Source: CAD feature listing. Evaluate the final solid. Frame: model axes, mm. Face numbers are marked on the shaded views. A direction names the side the tool comes from. Give positions to 0.01 mm unless a question says otherwise; leave off trailing zeros. Order: outer loops, then holes, each group sorted by start corner. A loop starts at its lowest first (then second) coordinate and runs counter-clockwise, first axis right, second up. Notation, with made-up numbers: (20, 88) - (28, 88) arc R14 ccw to (28, 95) - close; hole circle Ø1 at (15.25, 17.25). An arc over 180 degrees is marked (long way). Answer as CSV lines item,"result".
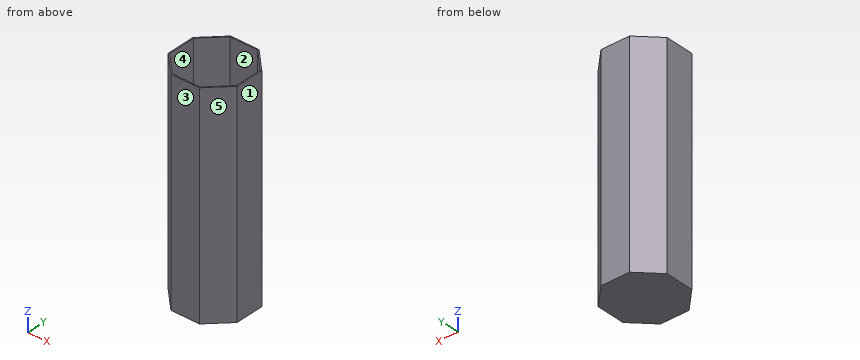
```python
from build123d import *

# Parameters (mm, degrees)
PAD006_DEPTH = 1
PAD005_DEPTH = 98


with BuildPart() as cooler_container_lid001:
    # Sketch007 → Pad006 (new body)
    with BuildSketch(Plane.XY):
        Polygon((15.9, 6.585996), (6.585996, 15.9), (-6.585996, 15.9), (-15.9, 6.585996), (-15.9, -6.585996), (-6.585996, -15.9), (6.585996, -15.9), (15.9, -6.585996), align=None)
    extrude(amount=PAD006_DEPTH)


with BuildPart() as cooler_walls_down:
    # Sketch006 → Pad005 (new body)
    with BuildSketch(Plane.XY):
        Polygon((15.9, 6.585996), (6.585996, 15.9), (-6.585996, 15.9), (-15.9, 6.585996), (-15.9, -6.585996), (-6.585996, -15.9), (6.585996, -15.9), (15.9, -6.585996), align=None)
        Polygon((15.4, 6.378889), (6.378889, 15.4), (-6.378889, 15.4), (-15.4, 6.378889), (-15.4, -6.378889), (-6.378889, -15.4), (6.378889, -15.4), (15.4, -6.378889), align=None, mode=Mode.SUBTRACT)
    extrude(amount=PAD005_DEPTH)


with BuildPart() as cooler_walls_down_1:
    # Body007 placement: moved
    add(cooler_walls_down.part.moved(Location((0, 0, 1))))

    # Fusion: union cooler_container_lid001
    add(cooler_container_lid001.part)


solid = cooler_walls_down_1.part
```
(1) Access query for the marked faces 4 and 5. Directions: +Z, -Z, +X, -X, +Y, -Y. A direction counts if a zero-diameter tool reaches every point of the face in a straight line with its end or side. Return the directions, or none.
Completed:
face 4,"+Z"
face 5,"+Z, -Z, +X, -Y"
(2) Cut plane A-A (z = 54.5). Return loops of the section in (x, y), then the cut area to 3 significant figures.
Completed:
outline,"(-15.9, -6.59) - (-6.59, -15.9) - (6.59, -15.9) - (15.9, -6.59) - (15.9, 6.59) - (6.59, 15.9) - (-6.59, 15.9) - (-15.9, 6.59) - close; hole (-15.4, -6.38) - (-6.38, -15.4) - (6.38, -15.4) - (15.4, -6.38) - (15.4, 6.38) - (6.38, 15.4) - (-6.38, 15.4) - (-15.4, 6.38) - close"
area,"51.9 mm²"
(3) Mould query, pull axis Y, two halves, no side actions, for the marked faces 1, 2 and 3. Classes: released by +Y, released by -Y, zero draft, split by the parting line, or undercut.
Completed:
face 1,"zero draft"
face 2,"undercut"
face 3,"released by -Y"
(4) Cut plane B-B (y = 3). Return loops of the section in (x, z), then the cut area to 3 significant figures.
Completed:
outline,"(-15.9, 0) - (15.9, 0) - (15.9, 99) - (15.4, 99) - (15.4, 1) - (-15.4, 1) - (-15.4, 99) - (-15.9, 99) - close"
area,"130 mm²"
(5) Contact query for flat-ended pins moving along their axis: pin 1 (2 mm diameter, centred on x = -9.5, z = 24.5, fed in from -Y); pin 2 (1 mm diameter, centred on x = 10, z = 31.5, fed in from -Y). Output: stop coordinate, or through.
Completed:
pin 1,"y = -13.99"
pin 2,"y = -12.99"
(6) Ray query, line 1 (Y direction, x = 5.5, z = 7); line 2 (Z direction, x = -3, y = -8). Return the intervals inside material, ascending. Write a range as from..to.
Completed:
line 1,"-15.9..-15.4, 15.4..15.9"
line 2,"0..1"
